Check sheet for the modelled part. Datum: model origin and axes. Units: mm. A direction names the side the tool comes from. Coordinates: 2 decimals unless noted, no trailing zeros. Order: outer loops, then holes, each group sorted by start corner. A loop starts at its lowest first (then second) coordinate and runs counter-clockwise, first axis right, second up. Notation, with made-up numbers: (32, 71) -> (66, 71) arc R18 cw to (66, 92) -> close; hole circle Ø4 at (14.25, 82). An arc over 180 degrees is marked (long way). Put each result on its own line as item: value. Start each with the question number.
```python
from build123d import *

# Parameters (mm, degrees)
SKETCH1_W                      = 100
SKETCH1_H                      = 100
BOSS_EXTRUDE1_DEPTH            = 15
SKETCH2_R                      = 40
CUT_EXTRUDE1_DEPTH             = 10.2
CUT_EXTRUDE2_REACH             = 73.443
SKETCH3_R                      = 30
CUT_EXTRUDE3_REACH             = 74.284
SKETCH4_W                      = 10.2
SKETCH4_H                      = 15
CUT_EXTRUDE3_DIRECTION_2_REACH = 74.284
CIRPATTERN1_COUNT              = 4
BOSS_EXTRUDE2_DEPTH            = 15
SKETCH6_W                      = 20.1
SKETCH6_H                      = 5
BOSS_EXTRUDE3_DEPTH            = 10
CIRPATTERN2_COUNT              = 4
CUT_EXTRUDE4_REACH             = 83.945
SKETCH7_R                      = 1.6
SKETCH8_R                      = 2.85
CUT_EXTRUDE5_DEPTH             = 2.5
CIRPATTERN3_COUNT              = 4
FILLET1_R                      = 2


with BuildPart() as part:
    # Sketch1 → Boss-Extrude1 (new body)
    with BuildSketch(Plane(origin=(0, 0, 0), x_dir=(1, 0, 0), z_dir=(0, 1, 0))):
        Rectangle(SKETCH1_W, SKETCH1_H)
    extrude(amount=BOSS_EXTRUDE1_DEPTH)

    # Sketch2 → Cut-Extrude1 (cut)
    with BuildSketch(Plane.XZ):
        with Locations(Location((0, 0, 0), (0, 0, 270))):
            Circle(SKETCH2_R)
    extrude(amount=-CUT_EXTRUDE1_DEPTH, mode=Mode.SUBTRACT)

    # Sketch3 → Cut-Extrude2 (cut, up to next)
    with BuildSketch(Plane.XZ.offset(-10.2), mode=Mode.PRIVATE) as cut_extrude2_sk1:
        with Locations(Location((0, 0, 0), (0, 0, 270))):
            Circle(SKETCH3_R)
    cut_extrude2_tool1 = extrude(cut_extrude2_sk1.sketch, amount=-CUT_EXTRUDE2_REACH, mode=Mode.PRIVATE) & part.part
    add(cut_extrude2_tool1.solids().sort_by_distance((0, 10.2, 0))[0], mode=Mode.SUBTRACT)

    # Sketch4 → Cut-Extrude3 (cut, up to next)
    with BuildSketch(Plane(origin=(0, 0, 0), x_dir=(-0.7071067811865475, 0, -0.7071067811865477), z_dir=(0.7071067811865477, 0, -0.7071067811865475)), mode=Mode.PRIVATE) as cut_extrude3_sk1:
        with Locations((-65.610678119, 7.5)):
            Rectangle(SKETCH4_W, SKETCH4_H)
    cut_extrude3_tool1 = extrude(cut_extrude3_sk1.sketch, amount=-CUT_EXTRUDE3_REACH, mode=Mode.PRIVATE) & part.part
    cut_extrude3 = cut_extrude3_tool1.solids().sort_by_distance((46.393755, 7.5, 46.393755))[0]
    add(cut_extrude3, mode=Mode.SUBTRACT)

    # Sketch4 → Cut-Extrude3 direction 2 (cut, up to next)
    with BuildSketch(Plane(origin=(0, 0, 0), x_dir=(-0.7071067811865475, 0, -0.7071067811865477), z_dir=(0.7071067811865477, 0, -0.7071067811865475)), mode=Mode.PRIVATE) as cut_extrude3_direction_2_sk1:
        with Locations((-65.610678119, 7.5)):
            Rectangle(SKETCH4_W, SKETCH4_H)
    cut_extrude3_direction_2_tool1 = extrude(cut_extrude3_direction_2_sk1.sketch, amount=CUT_EXTRUDE3_DIRECTION_2_REACH, mode=Mode.PRIVATE) & part.part
    cut_extrude3_direction_2 = cut_extrude3_direction_2_tool1.solids().sort_by_distance((46.393755, 7.5, 46.393755))[0]
    add(cut_extrude3_direction_2, mode=Mode.SUBTRACT)

    # CirPattern1: Cut-Extrude3, Cut-Extrude3 direction 2 ×4 about axis
    cirpattern1_axis = Axis((0, 0, 0), (0, 1, 0))
    add([cut_extrude3.rotate(cirpattern1_axis, i * 360 / CIRPATTERN1_COUNT) for i in range(1, CIRPATTERN1_COUNT)], mode=Mode.SUBTRACT)
    add([cut_extrude3_direction_2.rotate(cirpattern1_axis, i * 360 / CIRPATTERN1_COUNT) for i in range(1, CIRPATTERN1_COUNT)], mode=Mode.SUBTRACT)

    # Sketch5 → Boss-Extrude2 (add)
    with BuildSketch(Plane(origin=(0, 15, 0), x_dir=(1, 0, 0), z_dir=(0, 1, 0))):
        Polygon((-49.893933983, 35.681087681), (-53.429467889, 39.216621587), (-56.965001795, 35.681087681), (-50, 28.716085886), (-50, 35.575021664), align=None)
        Polygon((-39.216621587, 53.429467889), (-35.681087681, 56.965001795), (-28.716085886, 50), (-35.681087681, 49.893933983), align=None)
        Polygon((35.681087681, 49.893933983), (39.216621587, 53.429467889), (35.681087681, 56.965001795), (28.716085886, 50), align=None)
        Polygon((49.893933983, 35.681087681), (53.429467889, 39.216621587), (56.965001795, 35.681087681), (50, 28.716085886), align=None)
        Polygon((49.893933983, -35.681087681), (53.429467889, -39.216621587), (56.965001795, -35.681087681), (50, -28.716085886), align=None)
        Polygon((35.681087681, -49.893933983), (39.216621587, -53.429467889), (35.681087681, -56.965001795), (28.716085886, -50), align=None)
        Polygon((-35.681087681, -49.893933983), (-39.216621587, -53.429467889), (-35.681087681, -56.965001795), (-28.716085886, -50), align=None)
        Polygon((-49.893933983, -35.681087681), (-53.429467889, -39.216621587), (-56.965001795, -35.681087681), (-50, -28.716085886), align=None)
    extrude(amount=-BOSS_EXTRUDE2_DEPTH)

    # Sketch6 → Boss-Extrude3 (add)
    with BuildSketch(Plane(origin=(42.787510832, 0, 42.787510832), x_dir=(0.7071067811865476, 0, -0.7071067811865475), z_dir=(0.7071067811865475, 0, 0.7071067811865476))):
        with Locations((0, 12.5)):
            Rectangle(SKETCH6_W, SKETCH6_H)
    boss_extrude3 = extrude(amount=BOSS_EXTRUDE3_DEPTH)

    # CirPattern2: Boss-Extrude3 ×4 about axis
    cirpattern2_axis = Axis((0, 0, 0), (0, 1, 0))
    for i in range(1, CIRPATTERN2_COUNT):
        add(boss_extrude3.rotate(cirpattern2_axis, i * 360 / CIRPATTERN2_COUNT))

    # Sketch7 → Cut-Extrude4 (cut, up to next)
    with BuildSketch(Plane(origin=(0, 15, 0), x_dir=(1, 0, 0), z_dir=(0, 1, 0)), mode=Mode.PRIVATE) as cut_extrude4_sk1:
        with Locations(Location((44.696699141, 44.696699141, 0), (0, 0, 270))):
            Circle(SKETCH7_R)
    cut_extrude4_tool1 = extrude(cut_extrude4_sk1.sketch, amount=-CUT_EXTRUDE4_REACH, mode=Mode.PRIVATE) & part.part
    cut_extrude4 = cut_extrude4_tool1.solids().sort_by_distance((44.696699, 15, -44.696699))[0]
    add(cut_extrude4, mode=Mode.SUBTRACT)

    # Sketch8 → Cut-Extrude5 (cut)
    with BuildSketch(Plane(origin=(0, 15, 0), x_dir=(1, 0, 0), z_dir=(0, 1, 0))):
        with Locations(Location((44.696699141, 44.696699141, 0), (0, 0, 270))):
            Circle(SKETCH8_R)
    cut_extrude5 = extrude(amount=-CUT_EXTRUDE5_DEPTH, mode=Mode.SUBTRACT)

    # CirPattern3: Cut-Extrude4, Cut-Extrude5 ×4 about axis
    cirpattern3_axis = Axis((0, 0, 0), (0, 1, 0))
    add([cut_extrude4.rotate(cirpattern3_axis, i * 360 / CIRPATTERN3_COUNT) for i in range(1, CIRPATTERN3_COUNT)], mode=Mode.SUBTRACT)
    add([cut_extrude5.rotate(cirpattern3_axis, i * 360 / CIRPATTERN3_COUNT) for i in range(1, CIRPATTERN3_COUNT)], mode=Mode.SUBTRACT)

    # Fillet1
    fillet1_edges = [part.edges().sort_by_distance(p)[0] for p in [
        (32.198586784, 15, -53.482500897),
        (37.448854634, 15, -55.197234842),
        (35.681087681, 7.5, -56.965001795),
        (28.716085886, 7.5, -50),
        (53.482500897, 15, -32.198586784),
        (55.197234842, 15, -37.448854634),
        (50, 7.5, -28.716085886),
        (56.965001795, 7.5, -35.681087681),
        (55.197234842, 15, 37.448854634),
        (53.482500897, 15, 32.198586784),
        (56.965001795, 7.5, 35.681087681),
        (50, 7.5, 28.716085886),
        (32.198586784, 15, 53.482500897),
        (37.448854634, 15, 55.197234842),
        (28.716085886, 7.5, 50),
        (35.681087681, 7.5, 56.965001795),
        (39.216621587, 5, 53.429467889),
        (-37.448854634, 15, 55.197234842),
        (-32.198586784, 15, 53.482500897),
        (-35.681087681, 7.5, 56.965001795),
        (-28.716085886, 7.5, 50),
        (-53.482500897, 15, 32.198586784),
        (-55.197234842, 15, 37.448854634),
        (-50, 7.5, 28.716085886),
        (-56.965001795, 7.5, 35.681087681),
        (-55.197234842, 15, -37.448854634),
        (-53.482500897, 15, -32.198586784),
        (-50, 7.5, -28.716085886),
        (-56.965001795, 7.5, -35.681087681),
        (40.98438854, 15, 55.197234842),
        (55.197234842, 15, 40.98438854),
        (42.752155493, 12.5, 56.965001795),
        (56.965001795, 12.5, 42.752155493),
        (49.858578644, 15, 49.858578644),
        (55.197234842, 15, -40.98438854),
        (40.98438854, 15, -55.197234842),
        (56.965001795, 12.5, -42.752155493),
        (42.752155493, 12.5, -56.965001795),
        (49.858578644, 15, -49.858578644),
        (-40.98438854, 15, -55.197234842),
        (-55.197234842, 15, -40.98438854),
        (-42.752155493, 12.5, -56.965001795),
        (-56.965001795, 12.5, -42.752155493),
        (-49.858578644, 15, -49.858578644),
        (0, 15, 30),
        (-55.197234842, 15, 40.98438854),
        (-40.98438854, 15, 55.197234842),
        (-56.965001795, 12.5, 42.752155493),
        (-42.752155493, 12.5, 56.965001795),
        (-49.858578644, 15, 49.858578644),
        (0, 15, -50),
        (-50, 15, 0),
        (0, 15, 50),
        (50, 15, 0),
        (-32.198586784, 15, -53.482500897),
        (-37.448854634, 15, -55.197234842),
        (-28.716085886, 7.5, -50),
        (-35.681087681, 7.5, -56.965001795),
    ]]
    fillet(fillet1_edges, radius=FILLET1_R)


solid = part.part
```
1) Mould release check, pull along X, two halves, no side actions. Record for faces 4 (the flat face through (-50, 6, 0)), 5 (the cylindrical face through (-39.05, 5.03, 8.67)), 6 (the cylindrical face through (52.608, 14.43, 32.175)), 7 (the cylindrical face through (-38.02, 14.43, 53.775)): +X half, -X half, draft (parallel to the pull), parting line (faces both ways), or undercut.
2) Gauge pin test, flat ends, axial feed: pin 1 (8 mm diameter, centred on x = -2.5, y = 3.5, fed in from -Z); pin 2 (3.5 mm diameter, centred on x = -44.7, z = 44.7, fed in from +Y); pin 3 (6.5 mm diameter, centred on x = -5.5, y = 9.5, fed in from +Z); pin 4 (2.5 mm diameter, centred on x = -44.7, z = -44.7, fed in from -Y). Record the tip position at first contact, or that the pin passes through.
3) Sectioned sample at A-A (x = 0). Record the boundary of the cut face in (y, z).
4) Access from +Z, -Z, +X, -X, +Y, -Y to the whole of each face (thin tool, end or side, straight path). Record for faces 1 (the flat face through (-43, 12.5, 43)), 2 (the flat face through (-51.637, 5.07, -37.424)), 3 (the cylindrical face through (-53.775, 14.43, -38.02)).
5) Sectioned sample at B-B (z = 0). Record the boundary of the cut face in (x, y), plus the area to 3 significant figures.
6) Scan lines: line 1 along X through (y, z) = (6, -15); line 2 along X through (y, z) = (11.25, 0); line 3 along Z through (x, y) = (36, 0.5). Record each from-to range of solid material in increasing order. Write a range as [from, to].
Entries:
1. face 4: -X half
1. face 5: undercut
1. face 6: +X half
1. face 7: undercut
2. pin 1: stops at z = -50
2. pin 2: stops at y = 12.5
2. pin 3: stops at z = 50
2. pin 4: passes through
3. outline: (0, -50) -> (13, -50) arc R2 ccw to (15, -48) -> (15, -32) arc R2 ccw to (13, -30) -> (10.2, -30) -> (10.2, -40) -> (0, -40) -> close; (0, 40) -> (10.2, 40) -> (10.2, 30) -> (13, 30) arc R2 ccw to (15, 32) -> (15, 48) arc R2 ccw to (13, 50) -> (0, 50) -> close
4. face 1: +Y
4. face 2: -Z, -Y
4. face 3: -X, +Y
5. outline: (-50, 0) -> (-40, 0) -> (-40, 10.2) -> (-30, 10.2) -> (-30, 13) arc R2 ccw to (-32, 15) -> (-48, 15) arc R2 ccw to (-50, 13) -> close; (30, 10.2) -> (40, 10.2) -> (40, 0) -> (50, 0) -> (50, 13) arc R2 ccw to (48, 15) -> (32, 15) arc R2 ccw to (30, 13) -> close
5. area: 393 mm2
6. line 1: x = [-50, -37.08], [37.08, 50]
6. line 2: x = [-50, -30], [30, 50]
6. line 3: z = [-56.11, -50.21], [-49.58, -17.44], [17.44, 49.58], [50.21, 56.11]
